Source: CAD feature listing. Evaluate the final solid. Frame: model axes, mm. Coordinates: 2 decimals unless noted, no trailing zeros. Write each loop counter-clockwise with the first axis right and the second up, starting at its lowest first coordinate (ties: lowest second). Pieces come first, ordered by that corner, then holes. Notation, with made-up numbers: M 25.25,67.25 L 61.25,67.25 A18 cw 61.25,76.25 Z; hole C 58,50.5 d8. An arc over 180 degrees is marked long. Write item = value, one per line. Start each with the question number.
1. Section query B-B (x = -54.5). Output: boundary loops of the cut face in (y, z).
2. Line query: line 1 along Z through (x, y) = (-49.75, -2.75); line 2 along Z through (x, y) = (-46.75, -2.05); line 3 along Z through (x, y) = (-54, -1.65). Output: solid intervals per line, ascending.
3. Pull-direction query (X, two-part tool) for faces 1 (the face through (-58.718, -3, 29)), 2 (the face through (-48.452, -2.504, 52.192)), 3 (the face through (-50.024, -2.504, -9.763)); classes: pulls with the +X half, pulls with the -X half, needs draft (parallel to the pull), parting line crosses it, or undercut.
4. Pin query (flat end, axial travel): pin 1 Ø3 at (x, y) = (-54, -3.5) entering from +Z; pin 2 Ø1 at (x, y) = (-51.5, -2) entering from +Z; pin 3 Ø10 at (x, z) = (-48.5, 5.5) entering from +Y; pin 4 Ø6 at (x, z) = (-49.92, 0) entering from -Y. Return the tip coordinate at first contact, or that it passes through.
5. Section query A-A (z = 0). Output: boundary loops of the cut face in (x, y).
6. Section query C-C (y = -2.4). Output: boundary loops of the cut face in (x, z), then the cut area to 3 significant figures.
```python
from build123d import *

# Parameters (mm, degrees)
F1_DEPTH = 5.08
F3_D     = 7.62
F5_D     = 12.7


with BuildPart() as f1:
    # F0 (on Front) → F1 (new body)
    with BuildSketch(Plane.XZ):
        with BuildLine():
            ThreePointArc((-40.938293, 58.391372), (-49.828293, 67.281372), (-58.718293, 58.391372))
            Line((-58.718293, 58.391372), (-58.718293, -0.875289))
            ThreePointArc((-58.718293, -0.875289), (-49.828293, -9.765289), (-40.938293, -0.875289))
            Line((-40.938293, -0.875289), (-40.938293, 58.391372))
        make_face()
    extrude(amount=F1_DEPTH)

    # F3 (through all)
    with Locations(Plane(origin=(0, 0, 0), x_dir=(1, 0, 0), z_dir=(0, 1, 0))):
        with Locations((-49.923204, 0)):
            Hole(F3_D / 2)

    # F5 (through all)
    with Locations(Plane.XZ.offset(5.08)):
        with Locations((-49.828293, 58.391372)):
            Hole(F5_D / 2)


solid = f1.part
```
Results are:
q1.outline = M -5.08,-8.44 L 0,-8.44 L 0,54.09 L -5.08,54.09 Z; M -5.08,62.69 L 0,62.69 L 0,65.95 L -5.08,65.95 Z
q2.line_1 = -9.76 to -3.81, 3.81 to 52.04, 64.74 to 67.28
q2.line_2 = -9.22 to -2.11, 2.11 to 52.84, 63.95 to 66.73
q2.line_3 = -8.73 to 53.6, 63.18 to 66.24
q3.face_1 = pulls with the -X half
q3.face_2 = undercut
q3.face_3 = parting line crosses it
q4.pin_1 = 66.87
q4.pin_2 = 67.2
q4.pin_3 = 0
q4.pin_4 = through
q5.outline = M -58.72,-5.08 L -53.73,-5.08 L -53.73,0 L -58.72,0 Z; M -46.11,-5.08 L -40.94,-5.08 L -40.94,0 L -46.11,0 Z
q6.outline = M -58.72,-0.88 A8.89 ccw -40.94,-0.88 L -40.94,58.39 A8.89 ccw -58.72,58.39 Z; hole C -49.83,58.39 d12.7; hole C -49.92,0 d7.62
q6.area = 1,130 mm^2
